For this review, take the finished solid that the model builds, in its own axes (mm). A direction names the side the tool comes from. Give positions to 0.01 mm unless a question says otherwise; leave off trailing zeros. Write each loop counter-clockwise with the first axis right and the second up, starting at its lowest first coordinate (ties: lowest second). Pieces come first, ordered by that corner, then holes. Notation, with made-up numbers: (11.5, -28.5) -> (58.5, -28.5) arc R30 cw to (58.5, -4.5) -> close; hole circle Ø11 at (81, -20.75). An arc over 180 degrees is marked (long way). Write item = value, one per line.
```python
from build123d import *

# Parameters (mm, degrees)
ESQUISSE1_R             = 10
ESQUISSE1_R_2           = 5
BOSS_EXTRU_1_DEPTH      = 19
ENL_V_START             = -4
ESQUISSE2_W             = 20
ESQUISSE2_H             = 11
ENL_V_MAT_EXTRU_1_DEPTH = 39.249260349
ESQUISSE3_R             = 5
ENL_V_MAT_EXTRU_2_DEPTH = 43.249260349
BOSS_EXTRU_2_START      = 13
ESQUISSE4_R             = 9
ESQUISSE4_R_2           = 5
BOSS_EXTRU_2_DEPTH      = 13


with BuildPart() as part:
    # Esquisse1 → Boss.-Extru.1 (new body)
    # profile 1 of 2: a face of its own
    with BuildSketch(Plane.XY):
        with BuildLine():
            Line((0, 22), (0, 0))
            Line((0, 0), (20, 0))
            Line((20, 0), (20, 22))
            ThreePointArc((20, 22), (10, 12), (0, 22))
        make_face()
    # profile 2 of 2: a face of its own
    with BuildSketch(Plane.XY):
        with Locations((10, 22)):
            Circle(ESQUISSE1_R)
        with Locations((10, 22)):
            Circle(ESQUISSE1_R_2, mode=Mode.SUBTRACT)
    extrude(amount=BOSS_EXTRU_1_DEPTH)

    # Esquisse2 → Enlèv. mat.-Extru.1 (cut, through all)
    with BuildSketch(Plane.XZ.offset(ENL_V_START)):
        with Locations((10, 9.5)):
            Rectangle(ESQUISSE2_W, ESQUISSE2_H)
    extrude(amount=-ENL_V_MAT_EXTRU_1_DEPTH, mode=Mode.SUBTRACT)

    # Esquisse3 → Enlèv. mat.-Extru.2 (cut, through all)
    with BuildSketch(Plane.XZ):
        with Locations(Location((10, 9.5, 0), (0, 0, 270))):
            Circle(ESQUISSE3_R)
    extrude(amount=-ENL_V_MAT_EXTRU_2_DEPTH, mode=Mode.SUBTRACT)

    # Esquisse4 → Boss.-Extru.2 (add)
    with BuildSketch(Plane.XZ.offset(BOSS_EXTRU_2_START)):
        with Locations(Location((10, 9.5, 0), (0, 0, 270))):
            Circle(ESQUISSE4_R)
        with Locations(Location((10, 9.5, 0), (0, 0, 270))):
            Circle(ESQUISSE4_R_2, mode=Mode.SUBTRACT)
    extrude(amount=-BOSS_EXTRU_2_DEPTH)


solid = part.part
```
(1) Tool access review of faces 1 (the face through (10, 15, 4)), 2 (the face through (1.214, -6.591, 11.451)), 3 (the face through (11.5, -4.62, 4.73)): name each direction out of +Z, -Z, +X, -X, +Y, -Y from which nothing blocks a thin tool from reaching the whole face with its end or side.
Answers below:
face_1 = +X, -X, +Y
face_2 = -Y
face_3 = +Y, -Y
(2) Take a section at B-B (x = 10). Write out the cut boundary in (y, z).
Answers below:
outline = (-13, 0.5) -> (0, 0.5) -> (0, 0) -> (17, 0) -> (17, 4) -> (4, 4) -> (4, 4.5) -> (-13, 4.5) -> close; (-13, 14.5) -> (4, 14.5) -> (4, 15) -> (17, 15) -> (17, 19) -> (0, 19) -> (0, 18.5) -> (-13, 18.5) -> close; (27, 0) -> (32, 0) -> (32, 4) -> (27, 4) -> close; (27, 15) -> (32, 15) -> (32, 19) -> (27, 19) -> close
(3) Take a section at C-C (z = 9.5). Write out the cut boundary in (x, y).
Answers below:
outline = (0, 0) -> (1, 0) -> (1, -13) -> (5, -13) -> (5, 4) -> (0, 4) -> close; (15, -13) -> (19, -13) -> (19, 0) -> (20, 0) -> (20, 4) -> (15, 4) -> close
(4) To check wall thickness, follow probe 1 along X at (y, z) = (0.5, 9.5); probe 2 along Y at (x, z) = (9.75, 17); probe 3 along Z at (x, y) = (10.75, 13). State the ranges of each line that lie inside material, in increasing order.
Answers below:
probe_1 = 0 to 5, 15 to 20
probe_2 = -13 to 17.01, 26.99 to 32
probe_3 = 0 to 4, 15 to 19
(5) For pin 1 (3.5 mm diameter, centred on x = 6, z = 10.5, fed in from +Y); pin 2 (3 mm diameter, centred on x = 18, z = 15.5, fed in from +Y), all flat-tipped, find the tip position at first contact; note any pin that passes through.
Answers below:
pin_1 = 4
pin_2 = 29.6
(6) The part is to be moulded in two halves that separate along Y. For faces 4 (the face through (10.7, 0, 0.3)), 5 (the face through (10, 32, 17)), 6 (the face through (12.307, 17.564, 1.972)), say which applies: released by +Y, released by -Y, zero draft, split by the parting line, or undercut.
Answers below:
face_4 = released by -Y
face_5 = released by +Y
face_6 = undercut
(7) Take a section at A-A (y = 11.5). Write out the cut boundary in (x, z), plus the area to 3 significant figures.
Answers below:
outline = (0, 0) -> (20, 0) -> (20, 4) -> (0, 4) -> close; (0, 15) -> (20, 15) -> (20, 19) -> (0, 19) -> close
area = 160 mm^2
(8) Take a section at D-D (z = 3.5). Write out the cut boundary in (x, y), plus the area to 3 significant figures.
Answers below:
outline = (0, 0) -> (3.29, 0) -> (3.29, -13) -> (16.71, -13) -> (16.71, 0) -> (20, 0) -> (20, 22) arc R10 ccw to (0, 22) -> close; hole circle Ø10 at (10, 22)
area = 693 mm^2
